```python
from build123d import *

# Parameters (mm, degrees)
F0_W     = 110
F0_H     = 110
F0_W_2   = 69
F0_H_2   = 69
F1_DEPTH = 10
F2_DEPTH = 40


with BuildPart() as f1:
    # F0 (on Top) → F1 (new body)
    with BuildSketch(Plane.XY):
        with Locations((55, 55)):
            Rectangle(F0_W, F0_H)
        with Locations((55, 55)):
            Rectangle(F0_W_2, F0_H_2, mode=Mode.SUBTRACT)
    extrude(amount=F1_DEPTH)

    # F0 (on Top) → F2 (join)
    with BuildSketch(Plane.XY):
        with Locations((55, 55)):
            Rectangle(F0_W_2, F0_H_2)
    extrude(amount=F2_DEPTH)


solid = f1.part
```
Here's how the part is built. I have some questions about the finished solid (model axes, mm). A direction names the side the tool comes from. Give positions to 0.01 mm unless a question says otherwise; leave off trailing zeros. Order: outer loops, then holes, each group sorted by start corner. A loop starts at its lowest first (then second) coordinate and runs counter-clockwise, first axis right, second up. Notation, with made-up numbers: (37, -11.75) - (73, -11.75) arc R15 cw to (73, 16.25) - close; hole circle Ø2 at (2.5, 86.25). An arc over 180 degrees is marked (long way). Answer as a JSON object with one key per item and string values. Group by question number.
Item 1: For P1, Ø12, axis at x = 68, z = 32, coming from the -Y side; P2, Ø24, axis at y = 40, z = 32, coming from the +X side; P3, Ø15, axis at y = 60, z = 30.5, coming from the -X side, each with a flat end and sliding along its axis, tell me the tip position at first contact or that it passes through.
Item 2: Please list where these lines run through material, in increasing order: probe 1 along X at (y, z) = (39.5, 13.5); probe 2 along Z at (x, y) = (45.5, 93.5).
Item 3: If we section it at D-D on y = 10: Please give me the cut outline in (x, z).
Item 4: Which directions (+Z, -Z, +X, -X, +Y, -Y) give clear straight access to the entire face, cutting with the end or side of a thin tool? Please do faces 1 (the flat face through (55, 20.5, 25)), 2 (the flat face through (20.5, 55, 25)), 3 (the flat face through (55, 89.5, 25)), 4 (the flat face through (89.5, 55, 25)).
Item 5: If we section it at A-A on x = 45: Please give me the cut outline in (y, z), and give its area (3 significant figures).
Item 6: If we section it at C-C on z = 27: Please give me the cut outline in (x, y), and give its area (3 significant figures).
Result set:
{
 "1": {"P1": "y = 20.5", "P2": "x = 89.5", "P3": "x = 20.5"},
 "2": {"probe 1": "20.5 to 89.5", "probe 2": "0 to 10"},
 "3": {"outline": "(0, 0) - (110, 0) - (110, 10) - (0, 10) - close"},
 "4": {"face 1": "+Z, +X, -X, -Y", "face 2": "+Z, -X, +Y, -Y", "face 3": "+Z, +X, -X, +Y", "face 4": "+Z, +X, +Y, -Y"},
 "5": {"outline": "(0, 0) - (110, 0) - (110, 10) - (89.5, 10) - (89.5, 40) - (20.5, 40) - (20.5, 10) - (0, 10) - close", "area": "3,170 mm²"},
 "6": {"outline": "(20.5, 20.5) - (89.5, 20.5) - (89.5, 89.5) - (20.5, 89.5) - close", "area": "4,760 mm²"}
}
